Design review of the part built by this model. Coordinates are the model's own, in mm. A direction names the side the tool comes from. Coordinates: 2 decimals unless noted, no trailing zeros. Loops run counter-clockwise (first coordinate to the right, second up) from the corner with the lowest first, then second, coordinate; pieces in that order, holes last. Notation, with made-up numbers: (3.5, 79.25) - (45.5, 79.25) arc R19 ccw to (45.5, 107.25) - close; hole circle Ø4 at (53, -39). An arc over 180 degrees is marked (long way). Answer in a Markdown table with one row per item. Add a question column.
(1) To check wall thickness, follow L1, parallel to X at y = -62.5, z = -9.5; L2, parallel to Z at x = -195, y = -59; L3, parallel to Y at x = -68, z = 37. State the ranges of each line that lie inside material, in increasing order. Write a range as [from, to].
(2) Clearance check with flat-ended pins moving along their axes: pin 1 (14 mm diameter, centred on x = 7.5, y = -24, fed in from -Z); pin 2 (1.5 mm diameter, centred on x = -139, y = -45.5, fed in from -Z); pin 3 (14 mm diameter, centred on x = -262.5, z = 17, fed in from +Y). State where each tip first meets the part, or that it passes through.
(3) We need section D-D, the plane x = -235.5. Write out the cut boundary in (y, z).
(4) For faces 1 (the face through (-260.261, -13.768, 21.662)), 2 (the face through (6, -24, -15.51)), 3 (the face through (0, -24, 5)), 4 (the face through (-129, -23, 47.99)), list the 3-axis set-ups (+Z, -Z, +X, -X, +Y, -Y) from which the entire face can be reached by the end or side of a thin tool; tool diameter is ignored.
(5) We need section A-A, the plane z = -10.5. Write out the cut boundary in (x, y).
(6) We need section C-C, the plane y = -63. Write out the cut boundary in (x, z).
(7) The part is to be moulded in two halves that separate along Y. For faces 5 (the face through (-260.26, -32.91, 10.82)), 6 (the face through (-260, -23, 27.238)), 7 (the face through (-102, -67.787, 38)), 8 (the face through (-260, 20.993, 9)), say which applies: released by +Y, released by -Y, zero draft, split by the parting line, or undercut.
(8) We need section B-B, the plane z = 22.5. Write out the cut boundary in (x, y).
from build123d import *

# Parameters (mm, degrees)
F0_W     = 88.9
F0_H     = 63.5
F1_DEPTH = 12.7
F3_W     = 88.9880172908
F3_H     = 63.9023780823
F4_DEPTH = 12.7
F6_W     = 266.7
F6_H     = 88.9
F6_W_2   = 12.7
F7_DEPTH = 12.7
F8_DEPTH = 304.8


with BuildPart() as f1:
    # F0 (on Right) → F1 (new body)
    with BuildSketch(Plane.YZ):
        with Locations((-23.3373962309, 16.2396542728)):
            Rectangle(F0_W, F0_H)
    extrude(amount=F1_DEPTH)



with BuildPart() as f4:
    # F3 (on offset) → F4 (new body)
    with BuildSketch(Plane.YZ.offset(-254)):
        with Locations((-23.5012862831, 16.2396542728)):
            Rectangle(F3_W, F3_H)
    extrude(amount=-F4_DEPTH)


with BuildPart() as f1_1:
    add(f1.part)

    add(f4.part)  # F7 merges F4
    # F6 (on face) → F7 (join)
    with BuildSketch(Plane.XY.offset(47.9896542728)):
        with Locations((-133.35, -23.3373962309)):
            Rectangle(F6_W, F6_H)
        with Locations((6.35, -23.3373962309)):
            Rectangle(F6_W_2, F6_H)
    extrude(amount=-F7_DEPTH)

    # F5 (on face) → F8 (cut)
    with BuildSketch(Plane.YZ.offset(12.7)):
        Polygon((-16.9873962309, 5.2411316447), (-10.6373962309, 16.2396542728), (-16.9873962309, 27.2381769009), (-29.6873962309, 27.2381769009), (-36.0373962309, 16.2396542728), (-29.6873962309, 5.2411316447), align=None)
    extrude(amount=-F8_DEPTH, mode=Mode.SUBTRACT)


solid = f1_1.part
Responses:
| question | item | result |
|---|---|---|
| 1 | L1 | x = [-266.7, -254], [0, 12.7] |
| 1 | L2 | z = [35.29, 47.99] |
| 1 | L3 | y = [-67.79, 21.11] |
| 2 | pin 1 | stops at z = -15.51 |
| 2 | pin 2 | stops at z = 35.29 |
| 2 | pin 3 | stops at y = 20.99 |
| 3 | outline | (-67.79, 35.29) - (21.11, 35.29) - (21.11, 47.99) - (-67.79, 47.99) - close |
| 4 | face 1 | +X, -X |
| 4 | face 2 | -Z, +X, +Y, -Y |
| 4 | face 3 | -Z, +Y, -Y |
| 4 | face 4 | +Z, +X, +Y, -Y |
| 5 | outline | (-266.7, -68) - (-254, -68) - (-254, 20.99) - (-266.7, 20.99) - close; (0, -67.79) - (12.7, -67.79) - (12.7, 21.11) - (0, 21.11) - close |
| 6 | outline | (-266.7, -15.71) - (-254, -15.71) - (-254, 35.29) - (0, 35.29) - (0, -15.51) - (12.7, -15.51) - (12.7, 47.99) - (-254, 47.99) - (-254, 48.19) - (-266.7, 48.19) - close |
| 7 | face 5 | undercut |
| 7 | face 6 | undercut |
| 7 | face 7 | released by -Y |
| 7 | face 8 | released by +Y |
| 8 | outline | (-266.7, -68) - (-254, -68) - (-254, -32.42) - (-266.7, -32.42) - close; (-266.7, -14.25) - (-254, -14.25) - (-254, 20.99) - (-266.7, 20.99) - close; (0, -67.79) - (12.7, -67.79) - (12.7, -32.42) - (0, -32.42) - close; (0, -14.25) - (12.7, -14.25) - (12.7, 21.11) - (0, 21.11) - close |
